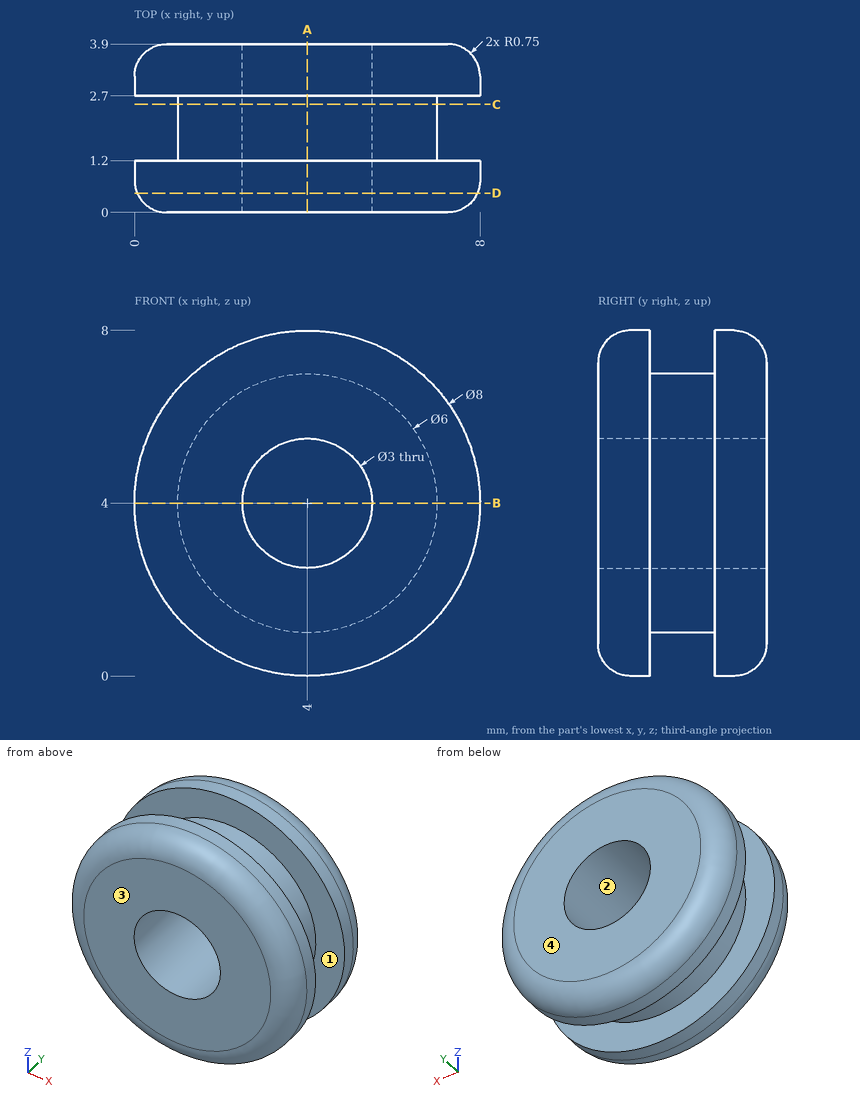
For this review, use the dimensioned drawing (mm, ordinates from the lowest corner) and the shaded views. Coordinates: 2 decimals unless noted, no trailing zeros. Write each loop counter-clockwise with the first axis right and the second up, starting at its lowest first coordinate (ties: lowest second). Pieces come first, ordered by that corner, then holes. Notation, with made-up numbers: (43.5, 66.5) - (54.5, 66.5) arc R26 cw to (54.5, 98.5) - close; hole circle Ø9 at (31, 22). An arc over 180 degrees is marked (long way). Answer as a JSON object with one key per item and string values. Group by question number.
1. Clearance check with flat-ended pins moving along their axes: pin 1 Ø1 at (x, z) = (7, 7) entering from -Y; pin 2 Ø2 at (y, z) = (2.5, 5.5) entering from +X; pin 3 Ø1.5 at (y, z) = (3, 2) entering from -X. State where each tip first meets the part, or that it passes through.
2. Add section B-B (z = 4). Give the boundary of the cut face in (x, y).
3. Add section D-D (y = 0.45). Give the boundary of the cut face in (x, z), plus the area to 3 significant figures.
4. To check wall thickness, follow probe 1 along X at (y, z) = (1.15, 4); probe 2 along X at (y, z) = (1.3, 4). State the ranges of each line that lie inside material, in increasing order.
5. Mouldability with a two-part tool opening along Y and no side actions: class the marked faces 1, 2, 3 and 4 as pulls with the +Y half, pulls with the -Y half, needs draft (parallel to the pull), parting line crosses it, or undercut.
6. Add section A-A (x = 4). Give the boundary of the cut face in (y, z), plus the area to 3 significant figures.
7. Add section C-C (y = 2.5). Give the boundary of the cut face in (x, z), plus the area to 3 significant figures.
Findings:
{
 "1": {"pin 1": "y = 0.18", "pin 2": "x = 7.97", "pin 3": "x = 0.2"},
 "2": {"outline": "(0, 0.75) arc R0.75 ccw to (0.75, 0) - (2.5, 0) - (2.5, 3.9) - (0.75, 3.9) arc R0.75 ccw to (0, 3.15) - (0, 2.7) - (1, 2.7) - (1, 1.2) - (0, 1.2) - close; (5.5, 0) - (7.25, 0) arc R0.75 ccw to (8, 0.75) - (8, 1.2) - (7, 1.2) - (7, 2.7) - (8, 2.7) - (8, 3.15) arc R0.75 ccw to (7.25, 3.9) - (5.5, 3.9) - close"},
 "3": {"outline": "circle Ø7.87 at (4, 4); hole circle Ø3 at (4, 4)", "area": "41.6 mm²"},
 "4": {"probe 1": "0 to 2.5, 5.5 to 8", "probe 2": "1 to 2.5, 5.5 to 7"},
 "5": {"face 1": "undercut", "face 2": "needs draft", "face 3": "pulls with the -Y half", "face 4": "pulls with the +Y half"},
 "6": {"outline": "(0, 0.75) arc R0.75 ccw to (0.75, 0) - (1.2, 0) - (1.2, 1) - (2.7, 1) - (2.7, 0) - (3.15, 0) arc R0.75 ccw to (3.9, 0.75) - (3.9, 2.5) - (0, 2.5) - close; (0, 5.5) - (3.9, 5.5) - (3.9, 7.25) arc R0.75 ccw to (3.15, 8) - (2.7, 8) - (2.7, 7) - (1.2, 7) - (1.2, 8) - (0.75, 8) arc R0.75 ccw to (0, 7.25) - close", "area": "16.0 mm²"},
 "7": {"outline": "circle Ø6 at (4, 4); hole circle Ø3 at (4, 4)", "area": "21.2 mm²"}
}
